The listing builds one solid part. Answer for the finished solid, in the listing's coordinates (mm). A direction names the side the tool comes from. Give positions to 0.01 mm unless a question says otherwise; leave off trailing zeros. Write each loop counter-clockwise with the first axis right and the second up, starting at its lowest first coordinate (ties: lowest second). Pieces come first, ordered by that corner, then holes. Notation, with made-up numbers: (18.25, 33) - (57.25, 33) arc R21 cw to (57.25, 70) - close; hole circle Ø9 at (85, -14.5). An arc over 180 degrees is marked (long way). Answer in a Markdown table with one row per item. Add a question column.
from build123d import *

# Parameters (mm, degrees)
CROQUIS1_R              = 2
SALIENTE_EXTRUIR1_DEPTH = 239


with BuildPart() as part:
    # Croquis1 → Saliente-Extruir1 (new body)
    with BuildSketch(Plane.XY):
        Polygon((-4.75, 10), (-10, 10), (-10, 4.75), (-8.25, 3), (-8.25, 5.5), (-6.5, 5.5), (-4, 3), (-4, -3), (-6.5, -5.5), (-8.25, -5.5), (-8.25, -3), (-10, -4.75), (-10, -10), (-4.75, -10), (-3, -8.25), (-5.5, -8.25), (-5.5, -6.5), (-3, -4), (3, -4), (5.5, -6.5), (5.5, -8.25), (3, -8.25), (4.75, -10), (10, -10), (10, -4.75), (8.25, -3), (8.25, -5.5), (6.5, -5.5), (4, -3), (4, 3), (6.5, 5.5), (8.25, 5.5), (8.25, 3), (10, 4.75), (10, 10), (4.75, 10), (3, 8.25), (5.5, 8.25), (5.5, 6.5), (3, 4), (-3, 4), (-5.5, 6.5), (-5.5, 8.25), (-3, 8.25), align=None)
        Circle(CROQUIS1_R, mode=Mode.SUBTRACT)
        Polygon((15.25, 10), (10, 10), (10, 4.75), (11.75, 3), (11.75, 5.5), (13.5, 5.5), (16, 3), (16, -3), (13.5, -5.5), (11.75, -5.5), (11.75, -3), (10, -4.75), (10, -10), (15.25, -10), (17, -8.25), (14.5, -8.25), (14.5, -6.5), (17, -4), (23, -4), (25.5, -6.5), (25.5, -8.25), (23, -8.25), (24.75, -10), (30, -10), (30, -4.75), (28.25, -3), (28.25, -5.5), (26.5, -5.5), (24, -3), (24, 3), (26.5, 5.5), (28.25, 5.5), (28.25, 3), (30, 4.75), (30, 10), (24.75, 10), (23, 8.25), (25.5, 8.25), (25.5, 6.5), (23, 4), (17, 4), (14.5, 6.5), (14.5, 8.25), (17, 8.25), align=None)
        with Locations((20, 0)):
            Circle(CROQUIS1_R, mode=Mode.SUBTRACT)
        Polygon((11.75, 3), (10, 4.75), (10, -4.75), (11.75, -3), (11.75, -5.5), (13.5, -5.5), (16, -3), (16, 3), (13.5, 5.5), (11.75, 5.5), align=None)
        Polygon((10, -4.75), (10, 4.75), (8.25, 3), (8.25, 5.5), (6.5, 5.5), (4, 3), (4, -3), (6.5, -5.5), (8.25, -5.5), (8.25, -3), align=None)
    extrude(amount=SALIENTE_EXTRUIR1_DEPTH)


solid = part.part
1. Section B-B (y = 0) is taken. Give the vertices of the cut face in (x, z), and give its area (3 significant figures).
2. Section C-C (z = 99.5) is taken. State how many separate pieces and enclosed holes the cut face has, and give its area (3 significant figures).
3. Given pin 1 Ø6.5 at (x, y) = (20, 0) entering from -Z; pin 2 Ø0.8 at (x, z) = (-4, 157.5) entering from +Y; pin 3 Ø1 at (y, z) = (-3.5, 115) entering from -X; pin 4 Ø3 at (x, z) = (21, 157) entering from -Y, each flat-ended and moving along its own axis, determine where each tip first touches the part or whether it passes through.
4. Straight lines are drawn through the part: L1, parallel to X at y = 0.25, z = 115; L2, parallel to X at y = -8, z = 10.5; L3, parallel to Y at x = 4, z = 35. For each, find the intervals that lie inside material, in ascending order. Write a range as [from, to].
5. Section A-A (x = 0) is taken. Give the vertices of the cut face in (y, z), and give its area (3 significant figures).
6. The mould has two halves that part along Y. Classify faces 5 (the face through (-7, -10, 118)), 6 (the face through (-4, 0, 118)), 7 (the face through (-7, 10, 118)): +Y half, -Y half, draft (parallel to the pull), parting line (faces both ways), or undercut.
7. A tool of negligible diameter and unlimited length cuts with its end or side. For faces 1 (the face through (20, -4, 118)), 2 (the face through (-10, -7, 118)), 3 (the face through (24, 0, 118)), 4 (the face through (0, 4, 118)), from which of +Z, -Z, +X, -X, +Y, -Y can it reach the whole face along a straight path? Write none if from no direction.
Geometry check:
| question | item | result |
|---|---|---|
| 1 | outline | (-4, 0) - (-2, 0) - (-2, 239) - (-4, 239) - close; (2, 0) - (18, 0) - (18, 239) - (2, 239) - close; (22, 0) - (24, 0) - (24, 239) - (22, 239) - close |
| 1 | area | 4,780 mm² |
| 2 | separate pieces | 1 |
| 2 | enclosed holes | 2 |
| 2 | area | 450 mm² |
| 3 | pin 1 | z = 0 |
| 3 | pin 2 | y = 9.65 |
| 3 | pin 3 | x = -9.25 |
| 3 | pin 4 | y = -4 |
| 4 | L1 | [-4, -1.98], [1.98, 18.02], [21.98, 24] |
| 4 | L2 | [-10, -5.5], [5.5, 14.5], [25.5, 30] |
| 4 | L3 | [-9.25, -8.25], [-5, 5], [8.25, 9.25] |
| 5 | outline | (-4, 0) - (-2, 0) - (-2, 239) - (-4, 239) - close; (2, 0) - (4, 0) - (4, 239) - (2, 239) - close |
| 5 | area | 956 mm² |
| 6 | face 5 | -Y half |
| 6 | face 6 | undercut |
| 6 | face 7 | +Y half |
| 7 | face 1 | +Z, -Z, -Y |
| 7 | face 2 | +Z, -Z, -X, +Y, -Y |
| 7 | face 3 | +Z, -Z, +X |
| 7 | face 4 | +Z, -Z, +Y |
